Source: three-view drawing plus pictorial views. Frame: mm from the lowest corner of the part. Coordinates: 2 decimals unless noted, no trailing zeros. Write each loop counter-clockwise with the first axis right and the second up, starting at its lowest first coordinate (ties: lowest second). Pieces come first, ordered by that corner, then holes. Notation, with made-up numbers: (36.5, 69) - (56.5, 69) arc R14 ccw to (56.5, 95) - close; hole circle Ø7 at (58.25, -17). An arc over 180 degrees is marked (long way). Put each result on its own line as item: value.
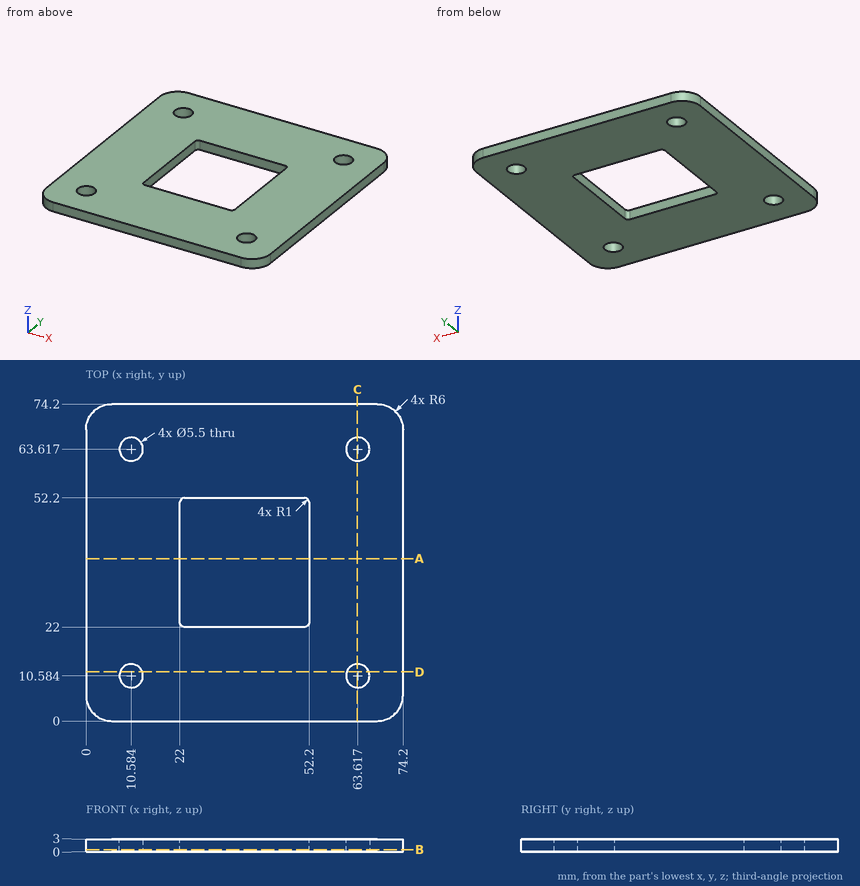
1. Pin query (flat end, axial travel): pin 1 Ø7 at (x, y) = (10.58, 63.62) entering from +Z. Return the tip coordinate at first contact, or that it passes through.
Answer below:
pin 1: stops at z = 3
2. Section query B-B (z = 0.5). Return loops of the section in (x, y), then the cut area to 3 significant figures.
Answer below:
outline: (0, 6) arc R6 ccw to (6, 0) - (68.2, 0) arc R6 ccw to (74.2, 6) - (74.2, 68.2) arc R6 ccw to (68.2, 74.2) - (6, 74.2) arc R6 ccw to (0, 68.2) - close; hole circle Ø5.5 at (10.58, 10.58); hole circle Ø5.5 at (10.58, 63.62); hole (22, 23) arc R1 ccw to (23, 22) - (51.2, 22) arc R1 ccw to (52.2, 23) - (52.2, 51.2) arc R1 ccw to (51.2, 52.2) - (23, 52.2) arc R1 ccw to (22, 51.2) - close; hole circle Ø5.5 at (63.62, 10.58); hole circle Ø5.5 at (63.62, 63.62)
area: 4,470 mm²
3. Section query D-D (y = 11.5). Return loops of the section in (x, z).
Answer below:
outline: (0, 0) - (7.99, 0) - (7.99, 3) - (0, 3) - close; (13.18, 0) - (61.02, 0) - (61.02, 3) - (13.18, 3) - close; (66.21, 0) - (74.2, 0) - (74.2, 3) - (66.21, 3) - close
4. Section query C-C (x = 63.5). Return loops of the section in (y, z) (1 decimal).
Answer below:
outline: (0, 0) - (7.8, 0) - (7.8, 3) - (0, 3) - close; (13.3, 0) - (60.9, 0) - (60.9, 3) - (13.3, 3) - close; (66.4, 0) - (74.2, 0) - (74.2, 3) - (66.4, 3) - close
5. Section query A-A (y = 38). Return loops of the section in (x, z), then the cut area to 3 significant figures.
Answer below:
outline: (0, 0) - (22, 0) - (22, 3) - (0, 3) - close; (52.2, 0) - (74.2, 0) - (74.2, 3) - (52.2, 3) - close
area: 132 mm²
6. Ray query, probe 1 along Y at (x, z) = (34, 0.7); probe 2 along Y at (x, z) = (10, 2.85) (1 decimal). Return the intervals inside material, ascending. Write a range as from..to.
Answer below:
probe 1: y = 0..22, 52.2..74.2
probe 2: y = 0..7.9, 13.3..60.9, 66.3..74.2
